Read the model definition and answer for the solid it produces. Units are mm, in the model's axes. Face numbers are marked on the shaded views. A direction names the side the tool comes from. Round coordinates to 2 decimals unless told otherwise and drop trailing zeros. Write each loop counter-clockwise with the first axis right and the second up, starting at its lowest first coordinate (ties: lowest second). Pieces come first, ordered by that corner, then holes. Notation, with made-up numbers: M -24.5,49 L 8.5,49 A31 ccw 8.5,85 Z; hole C 63.25,1.5 d7. An arc over 180 degrees is marked long. Use one line per item in the form item = value. Start each with the question number.
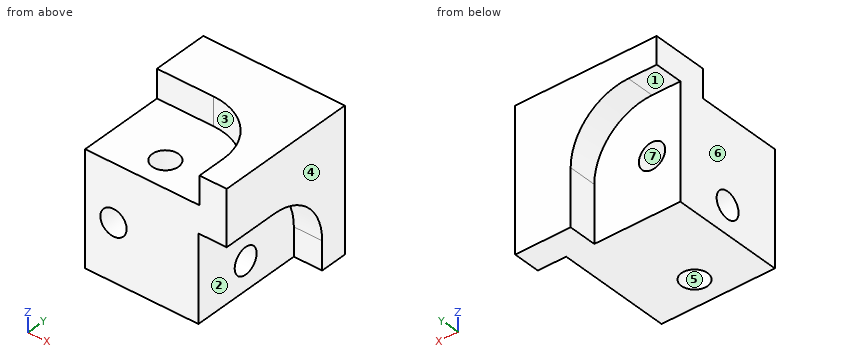
```python
from build123d import *

# Parameters (mm, degrees)
CUBE_BASE_DEPTH       = 7.9375
CUBE_BASE_DEPTH_BACK  = 7.9375
SKETCH2_W             = 15.875
SKETCH2_H             = 15.875
F_4_CLEARANCE_HOLE1_D = 2.9464
FRAME_RELIEF_DEPTH    = 3.175
CIRPATTERN1_COUNT     = 3


with BuildPart() as part:
    # Sketch2 → CUBE-BASE (new, two sides: drawn at the far end of the back side and taken through both)
    with BuildSketch(Plane.XY.offset(-CUBE_BASE_DEPTH_BACK)):
        Rectangle(SKETCH2_W, SKETCH2_H)
    extrude(amount=CUBE_BASE_DEPTH + CUBE_BASE_DEPTH_BACK)

    # 4 Clearance Hole1 (through all)
    with Locations(Plane.XY.offset(7.9375)):
        with Locations((-1.5875, -4.7625)):
            f_4_clearance_hole1 = Hole(F_4_CLEARANCE_HOLE1_D / 2)

    # Sketch5 → FRAME-RELIEF (cut)
    with BuildSketch(Plane.XY.offset(7.9375)):
        with BuildLine():
            Line((-1.5875, 1.7145), (-7.9375, 1.7145))
            Line((-7.9375, 1.7145), (-7.9375, -7.9375))
            Line((-7.9375, -7.9375), (4.8895, -7.9375))
            Line((4.8895, -7.9375), (4.8895, -4.7625))
            ThreePointArc((4.8895, -4.7625), (2.992430622, -0.182569378), (-1.5875, 1.7145))
        make_face()
    frame_relief = extrude(amount=-FRAME_RELIEF_DEPTH, mode=Mode.SUBTRACT)

    # CirPattern1: 4 Clearance Hole1, FRAME-RELIEF ×3 about axis
    cirpattern1_axis = Axis((0, 0, 0), (0.5773502691896253, 0.5773502691896268, 0.5773502691896253))
    add([f_4_clearance_hole1.rotate(cirpattern1_axis, i * 360 / CIRPATTERN1_COUNT) for i in range(1, CIRPATTERN1_COUNT)], mode=Mode.SUBTRACT)
    add([frame_relief.rotate(cirpattern1_axis, i * 360 / CIRPATTERN1_COUNT) for i in range(1, CIRPATTERN1_COUNT)], mode=Mode.SUBTRACT)


solid = part.part
```
Q1. For a pull along X with two mould halves and no side action, classify the marked faces 4, 5, 6 and 7 as +X half, -X half, draft (parallel to the pull), parting line (faces both ways), or undercut.
Q2. Each of these flat-tipped pins is pushed along its axis until it touches: pin 1 Ø2 at (y, z) = (3, -3) entering from +X; pin 2 Ø1 at (x, z) = (-4.5, 6.5) entering from -Y; pin 3 Ø5 at (x, y) = (-3, -4.5) entering from +Z. Where does it stop, or does it pass through?
Q3. Find section D-D on y = 4.25. Write down the section's boundary in (x, z).
Q4. Find section B-B on z = -6.5. Write down the section's boundary in (x, y), and give its area (3 significant figures).
Q5. A tool of negligible diameter and unlimited length cuts with its end or side. For the marked faces 1, 2 and 3, from which of +Z, -Z, +X, -X, +Y, -Y can it reach the whole face along a straight path? Write none if from no direction.
Q6. Find section C-C on x = -5. Write down the section's boundary in (y, z).
Q7. Straight lines are drawn through the part: line 1 (Z direction, x = 3.75, y = -1.5); line 2 (Z direction, x = -4, y = -2.75); line 3 (Z direction, x = 1, y = 0.5). For each, find the intervals that lie inside material, in ascending order. Write a range as [from, to].
Q8. Find section A-A on y = -3.75. Write down the section's boundary in (x, z), and give its area (3 significant figures).
Response:
q1.face_4 = +X half
q1.face_5 = undercut
q1.face_6 = -X half
q1.face_7 = undercut
q2.pin_1 = 4.76
q2.pin_2 = 1.71
q2.pin_3 = 4.76
q3.outline = M -7.94,-7.94 L 4.76,-7.94 L 4.76,-1.96 L 7.94,-1.96 L 7.94,7.94 L -7.94,7.94 Z; hole C -4.76,-1.59 d2.95
q4.outline = M -7.94,-7.94 L 4.76,-7.94 L 4.76,4.89 L 7.94,4.89 L 7.94,7.94 L 1.71,7.94 L 1.71,4.76 L -7.94,4.76 Z; hole C -1.59,-4.76 d2.95
q4.area = 174 mm²
q5.face_1 = -Z, -X, +Y
q5.face_2 = -Z, +X, -Y
q5.face_3 = +Z, -X, -Y
q6.outline = M -7.94,-7.94 L 4.76,-7.94 L 4.76,-3.04 L -7.94,-3.04 Z; M -7.94,-0.13 L 4.76,-0.13 L 4.76,4.89 L 7.94,4.89 L 7.94,7.94 L 1.71,7.94 L 1.71,4.76 L -7.94,4.76 Z; hole C -1.59,-4.76 d2.95
q7.line_1 = [-7.94, -6.23], [-3.29, 4.76]
q7.line_2 = [-7.94, -5.67], [-3.86, -2.85], [-0.33, 4.76]
q7.line_3 = [-7.94, 4.76]
q8.outline = M -7.94,-7.94 L -2.66,-7.94 L -2.66,4.76 L -7.94,4.76 Z; M -0.52,-7.94 L 4.76,-7.94 L 4.76,1.71 L 7.94,1.71 L 7.94,7.94 L 4.81,7.94 L 4.81,4.76 L -0.52,4.76 Z; hole C -4.76,-1.59 d2.95
q8.area = 147 mm²
